```python
from build123d import *

# Parameters (mm, degrees)
BOX002_W                  = 500
BOX002_H                  = 500
BOX002_DEPTH              = 500
BOX002_PLACEMENT_ANGLE    = 2
TUBE021_R                 = 85
TUBE021_R_2               = 80
TUBE021_DEPTH             = 19
TUBE013_R                 = 100
TUBE013_R_2               = 80
TUBE013_DEPTH             = 200
PAD028_DEPTH              = 100
PAD029_DEPTH              = 2
COMMON012_PLACEMENT_ANGLE = 38
ARRAY012_COUNT            = 22
ARRAY012_PLACEMENT_ANGLE  = 180
TUBE022_R                 = 34
TUBE022_R_2               = 30
TUBE022_DEPTH             = 19


with BuildPart() as cube002:
    # Box002 → Box002 (new body)
    with BuildSketch(Plane.XY):
        with Locations((250, 250)):
            Rectangle(BOX002_W, BOX002_H)
    extrude(amount=BOX002_DEPTH)


with BuildPart() as cube002_1:
    # Box002 placement: moved
    add(cube002.part.moved(Location((8.73, -250, 0))).rotate(Axis((8.73, -250, 0), (0, 0, 1)), BOX002_PLACEMENT_ANGLE))


with BuildPart() as tube021:
    # Tube021 → Tube021 (new body)
    with BuildSketch(Plane.XY.offset(100.5)):
        Circle(TUBE021_R)
        Circle(TUBE021_R_2, mode=Mode.SUBTRACT)
    extrude(amount=TUBE021_DEPTH)


with BuildPart() as tube013:
    # Tube013 → Tube013 (new body)
    with BuildSketch(Plane.XY):
        Circle(TUBE013_R)
        Circle(TUBE013_R_2, mode=Mode.SUBTRACT)
    extrude(amount=TUBE013_DEPTH)


with BuildPart() as body029:
    # Sketch028 → Pad028 (new body)
    with BuildSketch(Plane.XZ):
        Polygon((0, 0), (0, 2), (26, 0.9), (26, 0), align=None)
    extrude(amount=PAD028_DEPTH)


with BuildPart() as body029_1:
    # Body029 placement: moved
    add(body029.part.moved(Location((-5, 0, 5))))


with BuildPart() as cut002:
    # Sketch029 → Pad029 (new body)
    with BuildSketch(Plane.XY):
        Polygon((0, 0), (0, -52), (25.94305, -47.924315), (8.5, 0), align=None)
    extrude(amount=PAD029_DEPTH)


with BuildPart() as cut002_1:
    # Body030 placement: moved
    add(cut002.part.moved(Location((-5, -33, 5))))

    # Common012: intersect Body029
    add(body029_1.part, mode=Mode.INTERSECT)


with BuildPart() as cut002_2:
    # Common012 placement: moved
    add(cut002_1.part.rotate(Axis((0, 0, 0), (0, 1, 0)), COMMON012_PLACEMENT_ANGLE))

    # Array012: Cut002 ×22 about axis
    array012_axis = Axis((0, 0, 0), (0, 0, 1))


with BuildPart() as cut002_3:
    add(cut002_2.part)
    for i in range(1, ARRAY012_COUNT):
        add(cut002_2.part.rotate(array012_axis, i * 360 / ARRAY012_COUNT))


with BuildPart() as cut002_4:
    # Array012 placement: moved
    add(cut002_3.part.moved(Location((0, 0, 110))).rotate(Axis((0, 0, 110), (0, 1, 0)), ARRAY012_PLACEMENT_ANGLE))

    # Cut002: cut Tube013
    add(tube013.part, mode=Mode.SUBTRACT)


with BuildPart() as stator1h1:
    # Tube022 → Tube022 (new body)
    with BuildSketch(Plane.XY.offset(100.5)):
        Circle(TUBE022_R)
        Circle(TUBE022_R_2, mode=Mode.SUBTRACT)
    extrude(amount=TUBE022_DEPTH)

    # Fusion010: union Tube021, Cut002
    add(tube021.part)
    add(cut002_4.part)

    # Common017: intersect Cube002
    add(cube002_1.part, mode=Mode.INTERSECT)


solid = stator1h1.part
```
Can you work these out from the model? Positions are in its coordinate system, mm. A direction names the side the tool comes from. Give positions to 0.01 mm unless a question says otherwise; leave off trailing zeros. Loops run counter-clockwise (first coordinate to the right, second up) from the corner with the lowest first, then second, coordinate; pieces in that order, holes last. Notation, with made-up numbers: M 34.25,45 L 85.25,45 A34 cw 85.25,79 Z; hole C -23,19.25 d3. An arc over 180 degrees is marked long. One line per question, with ' | ' between items. Start each with the question number.
Q1. For faces 3 (the flat face through (26.883, -55.836, 107.541)), 4 (the flat face through (80, 7, 119.5)), 5 (the flat face through (60.014, -15.298, 108.813)), which set-ups out of +Z, -Z, +X, -X, +Y, -Y let a thin tool reach every point of the face, with its end or its side?
Q2. If we section it at A-A (y = 64): Please give me the cut outline in (x, z).
Q3. If we mould it in two halves opening along X, with no side actions, what happens to faces 1 (the flat face through (31, -2, 100.5)), 2 (the flat face through (42.997, -36.92, 102.205))? For each: +X half, -X half, draft (parallel to the pull), parting line (faces both ways), or undercut.
Q4. For pin 1 Ø1.5 at (x, z) = (57, 110.5) entering from -Y; pin 2 Ø8 at (x, y) = (21, -35.5) entering from -Z; pin 3 Ø8 at (y, z) = (13.5, 111.5) entering from +X, each with a flat end and sliding along its axis, tell me the tip position at first contact or that it passes through.
Q5. If I drill on line 1 (X direction, y = 50, z = 111.75); line 2 (Y direction, x = 6.5, z = 102.25); line 3 (X direction, y = 53, z = 104), over which ranges is the centre line in solid material (lowest first)? Write a range as from..to.
Computed:
1) face 3: -Z | face 4: +Z, +X, -X, +Y, -Y | face 5: +Z
2) outline: M -0.86,102.98 L 0.37,101.41 L 15.44,114.24 L 14.73,115.16 Z; M 17.89,102.98 L 19.18,101.41 L 37.16,116.11 L 36.43,116.88 Z; M 40.11,102.98 L 41.57,101.41 L 48,106.01 L 48,100.5 L 55.94,100.5 L 55.94,119.5 L 48,119.5 L 48,108.17 Z
3) face 1: draft | face 2: undercut
4) pin 1: stops at y = -63.73 | pin 2: stops at z = 101.41 | pin 3: stops at x = 84.47
5) line 1: x = 10.36..10.93, 25.48..27.72, 44.45..47.01, 62.45..68.74 | line 2: y = -84.75..-79.74, -33.37..-29.29, 29.29..33.37, 79.74..84.75 | line 3: x = 0.44..3.42, 16.02..19.12, 34.59..38.12, 59.92..66.45
